CAD build for the part. Positions are in the model's coordinates, mm. A direction names the side the tool comes from. Give positions to 0.01 mm unless a question says otherwise; leave off trailing zeros. Write each loop counter-clockwise with the first axis right and the second up, starting at its lowest first coordinate (ties: lowest second). Pieces come first, ordered by that corner, then holes. Notation, with made-up numbers: (-21, 46.25) -> (-14, 46.25) arc R28 ccw to (-14, 70.25) -> close; hole circle Ø4 at (27, 18.25). An arc over 180 degrees is marked (long way). Use one line per item in the form item = value. Start each with the question number.
from build123d import *

# Parameters (mm, degrees)
F0_W         = 29.62
F0_H         = 7.2
F1_DEPTH     = 6
F3_DEPTH     = 6
F5_DEPTH     = 6
F6_W         = 1
F6_H         = 6
F7_DEPTH     = 2.35
F8_W         = 3.025
F8_H         = 1.2
F9_DEPTH     = 9.191
F11_DEPTH    = 9.191
F12_W        = 0.625
F12_H        = 0.45
F13_DEPTH    = 9.191
F14_R        = 0.1
F16_DEPTH    = 3.84
F18_DEPTH    = 0.4
F20_DEPTH    = 6
F21_R        = 2.5
F22_DEPTH    = 3
F24_DEPTH    = 29.621
F25_T1_DEPTH = 7.5430097928
F25_T3_DEPTH = 7.5430097928
F27_DEPTH    = 6


# Not quite as in the source:
# - a fillet or chamfer that OpenCascade refuses, or shapes differently, is made with other operations: its cross-section is extruded or revolved along the edge and cut away or added


with BuildPart() as f1:
    # F0 (on Front) → F1 (new body)
    with BuildSketch(Plane.XZ):
        Rectangle(F0_W, F0_H)
    extrude(amount=-F1_DEPTH)

    # F2 (on face) → F3 (cut, through all)
    with BuildSketch(Plane.XZ):
        Polygon((10.97, -2.4), (14.81, -2.4), (14.81, 3.6), (4.67, 3.6), align=None)
    extrude(amount=-F3_DEPTH, mode=Mode.SUBTRACT)

    # F4 (on face) → F5 (cut, through all)
    with BuildSketch(Plane.XZ):
        Polygon((6.82, -3.6), (5.62, -2.4), (-14.81, -2.4), (-14.81, -3.6), align=None)
    extrude(amount=-F5_DEPTH, mode=Mode.SUBTRACT)

    # F6 (on face) → F7 (cut)
    with BuildSketch(Plane(origin=(0, 0, -2.4), x_dir=(1, 0, 0), z_dir=(0, 0, -1))):
        with Locations((0.69, -3)):
            Rectangle(F6_W, F6_H)
    extrude(amount=-F7_DEPTH, mode=Mode.SUBTRACT)

    # F8 (on face) → F9 (cut, through all)
    with BuildSketch(Plane.YZ.offset(14.81)):
        with Locations((4.4875, -3)):
            Rectangle(F8_W, F8_H)
    extrude(amount=-F9_DEPTH, mode=Mode.SUBTRACT)

    # F10 (on face) → F11 (cut, through all)
    with BuildSketch(Plane.YZ.offset(14.81)):
        Polygon((2.025, -3.6), (2.975, -3.6), (2.975, -2.4), align=None)
    extrude(amount=-F11_DEPTH, mode=Mode.SUBTRACT)

    # F12 (on face) → F13 (cut, through all)
    with BuildSketch(Plane.YZ.offset(14.81)):
        with Locations((0.3125, -3.375)):
            Rectangle(F12_W, F12_H)
        Polygon((0, -3.15), (0.625, -3.15), (1.625, -3.15), (1.625, -2.4), (0, -2.4), align=None)
    extrude(amount=-F13_DEPTH, mode=Mode.SUBTRACT)

    # F14
    f14_edges = [f1.edges().sort_by_distance(p)[0] for p in [
        (10.59, 1.625, -3.15),
    ]]
    fillet(f14_edges, radius=F14_R)

    # F15 (on face) → F16 (cut)
    with BuildSketch(Plane.YZ.offset(14.81)):
        Polygon((2.025, -2.7), (2.025, -3.6), (2.975, -2.4), (1.625, -2.4), (1.625, -2.7), align=None)
    extrude(amount=-F16_DEPTH, mode=Mode.SUBTRACT)

    # F17 (on face) → F18 (cut, through all)
    with BuildSketch(Plane.XZ.offset(-1.625)):
        Polygon((14.81, -2.8732050808), (14.81, -2.7), (14.71, -2.7), align=None)
    extrude(amount=-F18_DEPTH, mode=Mode.SUBTRACT)

    # F19 (on face) → F20 (cut, through all)
    with BuildSketch(Plane(origin=(0, 0, -2.4), x_dir=(1, 0, 0), z_dir=(0, 0, -1))):
        with BuildLine():
            ThreePointArc((-3.31, -3), (-5.8706601718, -1.9393398282), (-4.81, -4.5))
            ThreePointArc((-4.81, -4.5), (-3.7493398282, -4.0606601718), (-3.31, -3))
        make_face()
        with BuildLine():
            ThreePointArc((-9.31, -3), (-11.8706601718, -1.9393398282), (-10.81, -4.5))
            ThreePointArc((-10.81, -4.5), (-9.7493398282, -4.0606601718), (-9.31, -3))
        make_face()
    extrude(amount=-F20_DEPTH, mode=Mode.SUBTRACT)

    # F21 (on face) → F22 (cut)
    with BuildSketch(Plane(origin=(0, 0, -2.4), x_dir=(1, 0, 0), z_dir=(0, 0, -1))):
        with Locations((-10.81, -3)):
            Circle(F21_R)
        with Locations((-4.81, -3)):
            Circle(F21_R)
    extrude(amount=-F22_DEPTH, mode=Mode.SUBTRACT)

    # F23 (on face) → F24 (cut, through all)
    with BuildSketch(Plane(origin=(-14.81, 0, 0), x_dir=(0, -1, 0), z_dir=(-1, 0, 0))):
        with BuildLine():
            ThreePointArc((-5.79, -0.9), (-5.05, -1.64), (-4.31, -0.9))
            ThreePointArc((-4.31, -0.9), (-5.05, -0.16), (-5.79, -0.9))
        make_face()
    extrude(amount=-F24_DEPTH, mode=Mode.SUBTRACT)

    # F25: chamfer of 0.3 on 4 edges, made by hand

    # F25_s2 → F25_t1 (cut)
    with BuildSketch(Plane.XY.offset(-3.1715048964)):
        Polygon((-14.51, 0), (-14.81, 0.3), (-14.81, 0), align=None)
        Polygon((-14.51, 6), (-14.81, 5.7), (-14.81, 6), align=None)
    extrude(amount=F25_T1_DEPTH, mode=Mode.SUBTRACT)

    # F25_s4 → F25_t3 (cut)
    with BuildSketch(Plane.XZ.offset(-6.7715048964)):
        Polygon((-14.51, 3.6), (-14.81, 3.3), (-14.81, 3.6), align=None)
        Polygon((-14.81, -2.1), (-14.51, -2.4), (-14.81, -2.4), align=None)
    extrude(amount=F25_T3_DEPTH, mode=Mode.SUBTRACT)

    # F26 (on face) → F27 (cut, through all)
    with BuildSketch(Plane(origin=(0, 0, -2.4), x_dir=(1, 0, 0), z_dir=(0, 0, -1))):
        with BuildLine():
            ThreePointArc((4.19, -5.5), (5.2506601718, -5.0606601718), (5.69, -4))
            ThreePointArc((5.69, -4), (3.1293398282, -2.9393398282), (4.19, -5.5))
        make_face()
    extrude(amount=-F27_DEPTH, mode=Mode.SUBTRACT)


solid = f1.part
1) Wall check: line 1 along Y through (x, z) = (-4.81, -0.85); line 2 along X through (y, z) = (3, 2.15); line 3 along X through (y, z) = (1.45, 0). Give the ranges that are in metal, low to high. Write a range as from..to.
2) Cut at D-D (y = 5.05). State how many separate pieces and enclosed holes the cut face has, and give its area (3 significant figures).
3) 3-axis set-ups, long thin cutter, end or side, ignore diameter. For faces 4 (the face through (0.19, 3, -1)), 5 (the face through (-11.14, 0.52, -0.92)), 6 (the face through (11, 1, -3.15)): which of +Z, -Z, +X, -X, +Y, -Y reach the whole face in a straight line?
4) Cut at B-B (x = -5.25). Give the cut face in (y, z).
5) Cut at A-A (z = 1). Give the cut face in (x, y).
6) Pin check, flat tips, straight feed: pin 1 (1 mm diameter, centred on y = 3, z = 0, fed in from +X) (3 decimals); pin 2 (3 mm diameter, centred on y = 5, z = 1.5, fed in from +X); pin 3 (2.5 mm diameter, centred on x = -4.81, y = 3, fed in from +Z); pin 4 (0.7 mm diameter, centred on x = 11, y = 1, fed in from +Z). Stop position of each tip, or through.
7) Cut at C-C (z = -0.9). Give the cut face in (x, y) (3 decimals), and give its area (3 significant figures).
8) Two-plate mould, pull along Z, no slides. Class faces 1 (the face through (-14.81, 3, 1)), 2 (the face through (5.695, 5.637, -1.35)), 3 (the face through (6.23, 1.78, -3.01)): released by +Z, released by -Z, zero draft, split by the parting line, or undercut.
Final values:
q1.line_1 = 0..0.5, 5.79..6
q1.line_2 = -14.81..-12.31, -9.31..-6.31, -3.31..3.07, 5.31..6.19
q1.line_3 = -14.81..-12.77, -8.85..-6.77, -2.85..8.45
q2.separate_pieces = 7
q2.enclosed_holes = 0
q2.area = 80.8 mm^2
q3.face_4 = -Z, +Y, -Y
q3.face_5 = -Z
q3.face_6 = +X, -X, -Y
q4.outline = (0, -2.4) -> (0.54, -2.4) -> (0.54, 0.6) -> (1.57, 0.6) -> (1.57, 3.6) -> (0, 3.6) -> close; (4.43, 0.6) -> (5.46, 0.6) -> (5.46, -0.28) arc R0.74 cw to (5.46, -1.52) -> (5.46, -2.4) -> (6, -2.4) -> (6, 3.6) -> (4.43, 3.6) -> close
q5.outline = (-14.81, 0.3) -> (-14.51, 0) -> (7.4, 0) -> (7.4, 6) -> (-14.51, 6) -> (-14.81, 5.7) -> close; hole circle Ø3 at (-10.81, 3); hole circle Ø3 at (-4.81, 3); hole circle Ø3 at (4.19, 4)
q6.pin_1 = 8.975
q6.pin_2 = 8.45
q6.pin_3 = through
q6.pin_4 = -2.1
q7.outline = (-14.81, 0.3) -> (-14.51, 0) -> (0.19, 0) -> (0.19, 4.31) -> (-2.681, 4.31) arc R2.5 cw (long way) to (-6.939, 4.31) -> (-8.681, 4.31) arc R2.5 cw (long way) to (-12.939, 4.31) -> (-14.81, 4.31) -> close; (-14.72, 5.79) -> (0.19, 5.79) -> (0.19, 6) -> (-14.51, 6) -> close; (1.19, 0) -> (9.395, 0) -> (9.395, 4.31) -> (5.658, 4.31) arc R1.5 cw (long way) to (2.722, 4.31) -> (1.19, 4.31) -> close; (1.19, 5.79) -> (9.395, 5.79) -> (9.395, 6) -> (1.19, 6) -> close
q7.area = 68.2 mm^2
q8.face_1 = zero draft
q8.face_2 = undercut
q8.face_3 = released by -Z
